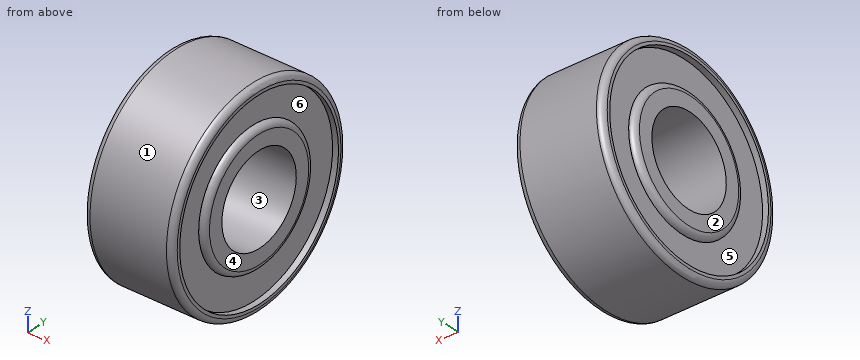
Autodesk Inventor part; units mm, degrees
ref_plane "YZ Plane" through (0, 0, 0) normal (1, 0, 0) x (0, 1, 0)
ref_plane "XZ Plane" through (0, 0, 0) normal (0, 1, 0) x (-1, 0, 0)
ref_plane "XY Plane" through (0, 0, 0) normal (0, 0, 1) x (1, 0, 0)
sketch "スケッチ1" plane through (0, 0, 0) normal (1, 0, 0) x (0, 1, 0)
  circle A0 centre (0, 0) radius 3.5
  dimension "d0" = 7
extrude "押し出し1" add sketch "スケッチ1" along normal blind 3
sketch "スケッチ2" plane through (3, 0, 0) normal (1, 0, 0) x (0, 0, -1)
  circle A0 centre (0, 0) radius 1.5
  dimension "d3" = 3
extrude "押し出し2" cut sketch "スケッチ2" against normal blind 3
sketch "スケッチ3" plane through (3, 0, 0) normal (1, 0, 0) x (0, 0, -1)
  circle A0 centre (0, 0) radius 3.2
  circle A1 centre (0, 0) radius 2.2
  circle A2 centre (0, 0) radius 3.5
  dimension "d6" = 0.3
  dimension "d7" = 1
extrude "押し出し3" cut sketch "スケッチ3" against normal blind 0.2 contours A0
sketch "スケッチ4" plane through (0, 0, 0) normal (-1, 0, 0) x (0, 0, 1)
  circle A0 centre (0, 0) radius 3.2
  circle A1 centre (0, 0) radius 2.2
extrude "押し出し4" cut sketch "スケッチ4" against normal blind 0.2
fillet "フィレット1" radius 0.2 4 edges at (0, -3.5, 0) (0, 0, -2.2) (3, -3.5, 0) (3, 0, 2.2)
properties part number "bearing" material "鋼、合金"
Work out the finished part from the listing and answer in its coordinate system (mm). Face numbers are marked on the shaded views. A direction names the side the tool comes from. Give positions to 0.01 mm unless a question says otherwise; leave off trailing zeros. Order: outer loops, then holes, each group sorted by start corner. A loop starts at its lowest first (then second) coordinate and runs counter-clockwise, first axis right, second up. Notation, with made-up numbers: M 19,-29 L 32,-29 A10 ccw 32,-17 Z; hole C -1,27 d9. An arc over 180 degrees is marked long. Return JSON: item names as keys, results as strings.
Q1. The mould has two halves that part along Y. Classify the marked faces 1, 2 and 3: pulls with the +Y half, pulls with the -Y half, needs draft (parallel to the pull), parting line crosses it, or undercut.
Answer below:
{"face 1": "parting line crosses it", "face 2": "needs draft", "face 3": "undercut"}
Q2. Find the intervals of material crossed by line 1 along X through (y, z) = (0.5, 2.75); line 2 along Y through (x, z) = (2.85, 2.75); line 3 along Z through (x, y) = (0.75, 2.5), in increasing order. Write a range as [from, to].
Answer below:
{"line 1": "x = [0.2, 2.8]", "line 2": "y = [-2.15, -1.64], [1.64, 2.15]", "line 3": "z = [-2.45, 2.45]"}
Q3. Each of these flat-tipped pins is pushed along its axis until it touches: pin 1 (1.5 mm diameter, centred on x = 1, y = -1.5, fed in from -Z); pin 2 (1.5 mm diameter, centred on x = 2, y = 3, fed in from -Z). Where does it stop, or does it pass through?
Answer below:
{"pin 1": "stops at z = -3.42", "pin 2": "stops at z = -2.68"}
Q4. Find section C-C, the plane x = 2.4. Write down the section's boundary in (y, z).
Answer below:
{"outline": "C 0,0 d7; hole C 0,0 d3"}
Q5. Which of the six approach directions +Z, -Z, +X, -X, +Y, -Y give full straight-line access (tool end or side, diameter ignored) to the marked faces 4, 5 and 6?
Answer below:
{"face 4": "+Z, -Z, +X, +Y, -Y", "face 5": "-X", "face 6": "+X"}
